The listing builds one solid part. Answer for the finished solid, in the listing's coordinates (mm). Round coordinates to 2 decimals unless told otherwise and drop trailing zeros. Order: outer loops, then holes, each group sorted by start corner. A loop starts at its lowest first (then second) coordinate and runs counter-clockwise, first axis right, second up. Notation, with made-up numbers: (-11.5, 1.25) -> (45.5, 1.25) arc R24 ccw to (45.5, 38.25) -> close; hole circle Ø5 at (24, 24.5). An arc over 180 degrees is marked (long way). Answer in a Markdown table with one row per item. Add a question column.
Autodesk Inventor part; units mm, degrees
ref_plane "YZ Plane" through (0, 0, 0) normal (1, 0, 0) x (0, 1, 0)
ref_plane "XZ Plane" through (0, 0, 0) normal (0, 1, 0) x (-1, 0, 0)
ref_plane "XY Plane" through (0, 0, 0) normal (0, 0, 1) x (1, 0, 0)
sketch "Sketch1" plane through (0, 0, 0) normal (0, 0, 1) x (1, 0, 0)
  arc A0 (51.4063, 79.344) -> (51.4063, -79.344) centre (0, 0) ccw
  arc A1 (167.2707, -4.2764) -> (167.2707, 4.2764) centre (164.5, 0) ccw
  line L0 (51.4063, 79.344) -> (167.2707, 4.2764)
  line L1 (167.2707, -4.2764) -> (51.4063, -79.344)
  line L2 (-150.1688, 0) -> (225.2229, 0)
  arc A2 (52.4938, 81.0225) -> (52.4938, -81.0225) centre (0, 0) ccw
  arc A3 (168.3582, -5.9549) -> (168.3582, 5.9549) centre (164.5, 0) ccw
  line L3 (52.4938, 81.0225) -> (168.3582, 5.9549)
  line L4 (168.3582, -5.9549) -> (52.4938, -81.0225)
  dimension "d0" = 2
  dimension "d2" = 5.0955
  dimension "d5" = 94.5414
  dimension "d6" = 164.5
extrude "Extrusion1" add sketch "Sketch1" along normal blind 6 contours A0 L2 A2 L3 A3 A1 L0 | A0 L1 A1 L2 A3 L4 A2
properties part number "belt"
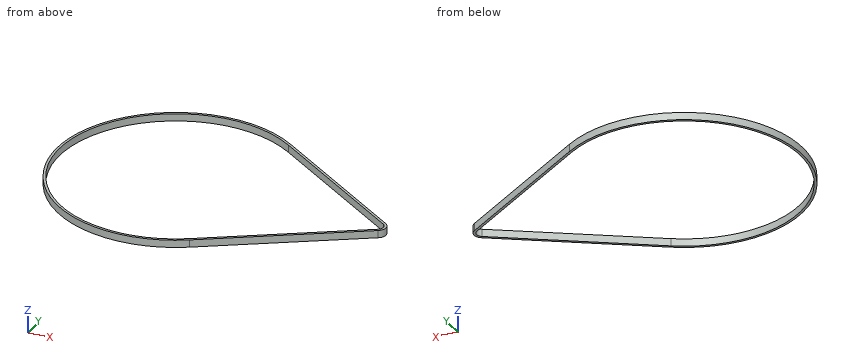
1. Straight lines are drawn through the part: line 1 along X through (y, z) = (0, 2.1); line 2 along Y through (x, z) = (0, 3.35); line 3 along X through (y, z) = (79.5, 4). For each, find the intervals that lie inside material, in ascending order.
2. The part is cut by section A-A (x = 0). Give the vertices of the cut face in (y, z).
3. The part is cut by section B-B (y = 0). Give the vertices of the cut face in (x, z).
4. Each of these flat-tipped pins is pushed along its axis until it touches: pin 1 (1 mm diameter, centred on x = 133.5, z = 1.5, fed in from +Y); pin 2 (3 mm diameter, centred on x = 70, z = 1, fed in from +Y). Where does it stop, or does it pass through?
5. The part is cut by section C-C (z = 4.8). Give the vertices of the cut face in (x, y).
Report:
| question | item | result |
|---|---|---|
| 1 | line 1 | x = -96.54 to -94.54, 169.6 to 171.6 |
| 1 | line 2 | y = -96.54 to -94.54, 94.54 to 96.54 |
| 1 | line 3 | x = -54.77 to -51.16, 51.16 to 54.84 |
| 2 | outline | (-96.54, 0) -> (-94.54, 0) -> (-94.54, 6) -> (-96.54, 6) -> close; (94.54, 0) -> (96.54, 0) -> (96.54, 6) -> (94.54, 6) -> close |
| 3 | outline | (-96.54, 0) -> (-94.54, 0) -> (-94.54, 6) -> (-96.54, 6) -> close; (169.6, 0) -> (171.6, 0) -> (171.6, 6) -> (169.6, 6) -> close |
| 4 | pin 1 | stops at y = 28.86 |
| 4 | pin 2 | stops at y = 70.65 |
| 5 | outline | (52.49, -81.02) -> (168.36, -5.95) arc R7.1 ccw to (168.36, 5.95) -> (52.49, 81.02) arc R96.54 ccw (long way) to start; hole (51.41, -79.34) -> (167.27, -4.28) arc R5.1 ccw to (167.27, 4.28) -> (51.41, 79.34) arc R94.54 ccw (long way) to start |
